The listing builds one solid part. Answer for the finished solid, in the listing's coordinates (mm). A direction names the side the tool comes from. Give positions to 0.01 mm unless a question says otherwise; leave off trailing zeros. Write each loop counter-clockwise with the first axis right and the second up, starting at its lowest first coordinate (ties: lowest second). Pieces come first, ordered by that corner, then holes. Notation, with made-up numbers: (3, 14) -> (50, 14) arc R35 cw to (50, 46) -> close; hole circle Ø3 at (-32, 86.5). An arc over 180 degrees is marked (long way). Put each result on its own line as item: value. Start each with the question number.
1) For faces 4 (the cylindrical face through (4.444, 18.544, -35.863)), 5 (the flat face through (0, 18, 50.8)), determine the directions among +Z, -Z, +X, -X, +Y, -Y from which every point of the face is accessible in a straight line to the end or side of a thin tool.
2) A cutting plane is placed at A-A (y = 20.5). Write down the section's boundary in (x, z) (3 decimals).
3) A cutting plane is placed at B-B (z = -36). Write down the section's boundary in (x, y).
4) A cutting plane is placed at D-D (z = 36.5). Write down the section's boundary in (x, y), then the cut area to 3 significant figures.
5) Find the intervals of material crossed by line 1 along Z through (x, y) = (-0.75, 27); line 2 along Z through (x, y) = (1, 2.5); line 3 along X through (y, z) = (7, -36.5), in increasing order. Write a range as from..to.
6) For a pull along X with two mould halves and no side action, classify faces 1 (the cylindrical face through (4.444, 18.544, 36.019)), 2 (the flat face through (12.7, 18, -1)), 3 (the flat face through (0, 36.576, 1)) as released by +X, released by -X, zero draft, split by the parting line, or undercut.
7) A cutting plane is placed at C-C (x = 3.5). Write down the section's boundary in (y, z).
from build123d import *

# Parameters (mm, degrees)
F0_W     = 25.4
F0_H     = 101.6
F1_DEPTH = 36.576
F2_D     = 8.89
F3_D     = 9.7282


with BuildPart() as f1:
    # F0 (on Front) → F1 (new body)
    with BuildSketch(Plane.XZ):
        Rectangle(F0_W, F0_H)
    extrude(amount=-F1_DEPTH)

    # F2 (through all)
    with Locations(Plane.XZ):
        with Locations((0, 35.941), (0, -35.941)):
            Hole(F2_D / 2)

    # F3 (through all)
    with Locations(Plane.XZ):
        with Locations((-1.016, 35.941), (-1.016, -35.941)):
            Hole(F3_D / 2)


solid = f1.part
Reply:
1. face 4: +Y, -Y
1. face 5: +Z, +X, -X, +Y, -Y
2. outline: (-12.7, -50.8) -> (12.7, -50.8) -> (12.7, 50.8) -> (-12.7, 50.8) -> close; hole (1.412, -40.156) arc R4.445 ccw to (1.412, -31.726) arc R4.864 ccw (long way) to start; hole (1.412, 31.726) arc R4.445 ccw to (1.412, 40.156) arc R4.864 ccw (long way) to start
3. outline: (-12.7, 0) -> (-5.88, 0) -> (-5.88, 36.58) -> (-12.7, 36.58) -> close; (4.44, 0) -> (12.7, 0) -> (12.7, 36.58) -> (4.44, 36.58) -> close
4. outline: (-12.7, 0) -> (-5.85, 0) -> (-5.85, 36.58) -> (-12.7, 36.58) -> close; (4.41, 0) -> (12.7, 0) -> (12.7, 36.58) -> (4.41, 36.58) -> close
4. area: 554 mm2
5. line 1: z = -50.8..-40.8, -31.08..31.08, 40.8..50.8
5. line 2: z = -50.8..-40.37, -31.51..31.51, 40.37..50.8
5. line 3: x = -12.7..-5.85, 4.41..12.7
6. face 1: undercut
6. face 2: released by +X
6. face 3: zero draft
7. outline: (0, -50.8) -> (36.58, -50.8) -> (36.58, -38.68) -> (0, -38.68) -> close; (0, -33.2) -> (36.58, -33.2) -> (36.58, 33.2) -> (0, 33.2) -> close; (0, 38.68) -> (36.58, 38.68) -> (36.58, 50.8) -> (0, 50.8) -> close
